Autodesk Inventor part; units mm, degrees
ref_plane "YZ Plane" through (0, 0, 0) normal (1, 0, 0) x (0, 1, 0)
ref_plane "XZ Plane" through (0, 0, 0) normal (0, 1, 0) x (-1, 0, 0)
ref_plane "XY Plane" through (0, 0, 0) normal (0, 0, 1) x (1, 0, 0)
sketch "Skizze1" plane through (0, 0, 0) normal (0, 0, 1) x (1, 0, 0)
  line L0 (-3.175, -3.175) -> (3.175, -3.175)
  line L1 (3.175, -3.175) -> (3.175, 3.175)
  line L2 (3.175, 3.175) -> (-3.175, 3.175)
  line L3 (-3.175, 3.175) -> (-3.175, -3.175)
  line L4 (-3.175, -3.175) -> (3.175, 3.175) construction
  line L5 (3.175, -3.175) -> (-3.175, 3.175) construction
  point P0 (0, 0)
  dimension "d0" = 6.35
  dimension "d1" = 6.35
extrude "Extrusion1" add sketch "Skizze1" along normal blind 1.65
sketch "Skizze2" plane through (0, 0, 1.65) normal (0, 0, 1) x (1, 0, 0)
  circle A0 centre (0, 0) radius 3.175
  dimension "d4" = 6.35
extrude "Extrusion2" add sketch "Skizze2" along normal blind 7.87
sketch "Skizze3" plane through (0, 0, 9.52) normal (0, 0, 1) x (1, 0, 0)
  circle A0 centre (0, 0) radius 2.155
  dimension "d7" = 4.31
extrude "Extrusion3" cut sketch "Skizze3" against normal blind 2
sketch "Skizze4" plane through (0, 0, 7.52) normal (0, 0, 1) x (1, 0, 0)
  circle A0 centre (0, 0) radius 0.38
  dimension "d10" = 0.76
extrude "Extrusion4" cut sketch "Skizze4" against normal blind 5
thread "Gewinde1"
sketch "Skizze5" plane through (0, 0, 0) normal (0, 0, -1) x (-1, 0, 0)
  circle A0 centre (0, 0) radius 0.5
  dimension "d15" = 1
extrude "Extrusion5" add sketch "Skizze5" along normal blind 3.81
sketch "Skizze6" plane through (0, 0, 0) normal (0, 0, -1) x (-1, 0, 0)
  line L0 (0, -4.445) -> (0, 4.445)
  line L1 (3.175, 3.175) -> (3.175, 0)
  arc A0 (-3.175, 0) -> (0, -3.175) centre (0, 0) ccw
  line L2 (3.175, 3.175) -> (2.105, 3.175)
  line L3 (2.105, 3.175) -> (2.105, 2.105)
  line L4 (2.105, 2.105) -> (3.175, 2.105)
  line L5 (3.175, 2.105) -> (3.175, 3.175)
  line L6 (-3.175, 3.175) -> (-2.105, 3.175)
  line L7 (-2.105, 3.175) -> (-2.105, 2.105)
  line L8 (-2.105, 2.105) -> (-3.175, 2.105)
  line L9 (-3.175, 2.105) -> (-3.175, 3.175)
  line L10 (-3.175, 3.175) -> (3.175, 3.175)
  line L11 (3.175, 0.375) -> (2.155, 0.375)
  line L12 (2.155, 0.375) -> (2.155, -0.645)
  line L13 (2.155, -0.645) -> (3.175, -0.645)
  line L14 (3.175, -0.645) -> (3.175, 0.375)
  line L15 (-3.175, -3.175) -> (-3.175, 3.175)
  line L16 (-3.175, 0.375) -> (-2.155, 0.375)
  line L17 (-2.155, 0.375) -> (-2.155, -0.645)
  line L18 (-2.155, -0.645) -> (-3.175, -0.645)
  line L19 (-3.175, -0.645) -> (-3.175, 0.375)
  dimension "d22" = 1.07
  dimension "d23" = 1.07
  dimension "d24" = 1.07
  dimension "d25" = 1.07
  dimension "d28" = 1.02
  dimension "d29" = 1.02
  dimension "d30" = 1.02
  dimension "d31" = 1.02
  dimension "d32" = 1.73
extrude "Extrusion6" add sketch "Skizze6" along normal blind 3.81 contours L1 L14 L13 L12 L11 | L2 L1 L4 L3 | L18 L15 A0 | A0 L15 L16 L17 L18 | L7 L8 L9 L6
properties part number "CON-SMA-EDGE-S" material "Messing, weicher Gelbton"
Check sheet for the modelled part. Datum: model origin and axes. Units: mm. A direction names the side the tool comes from. Round coordinates to 2 decimals unless told otherwise and drop trailing zeros. Loops run counter-clockwise (first coordinate to the right, second up) from the corner with the lowest first, then second, coordinate; pieces in that order, holes last. Notation, with made-up numbers: M 48.5,63.5 L 83.5,63.5 A6 ccw 83.5,73.5 Z; hole C 43.25,41.5 d8. An arc over 180 degrees is marked long. One line per question, with ' | ' between items. Start each with the question number.
Item 1: Section check A-A (z = -2.5). Record the boundary of the cut face in (x, y) (3 decimals), and give its area (3 significant figures).
Item 2: Section check C-C (x = -1). Record the boundary of the cut face in (y, z) (3 decimals), and give its area (3 significant figures).
Item 3: Section check D-D (z = 5.5). Record the boundary of the cut face in (x, y) (3 decimals).
Item 4: Gauge pin test, flat ends, axial feed: pin 1 Ø0.9 at (x, z) = (2.5, -3) entering from -Y (3 decimals); pin 2 Ø3.5 at (x, y) = (1, -1.5) entering from +Z. Record the tip position at first contact, or that the pin passes through.
Item 5: Scan lines: probe 1 along Y at (x, z) = (0, 4.9) (3 decimals); probe 2 along Y at (x, z) = (0, 8.25) (3 decimals); probe 3 along Z at (x, y) = (-1, 1.25). Record each from-to range of solid material in increasing order.
Item 6: Section check B-B (y = 0.75). Record the boundary of the cut face in (x, z) (3 decimals).
Item 7: Set-up check for faces 1 (the face through (3, 0.375, -2)), 2 (the face through (3, -3, 1.65)), 3 (the face through (-1.71, -1.31, 8.53)), 4 (the face through (-3, -2, 1.65)), 5 (the face through (3, 2.105, -2)): record each of +Z, -Z, +X, -X, +Y, -Y from which the full face is reachable in a straight line by a thin tool's end or side.
Item 8: Release check for a two-part mould opening along X. For faces 6 (the face through (0.108, 0.488, -1.878)), 7 (the face through (-3.175, 0, -1)), 8 (the face through (-3, 2.105, -2)), 9 (the face through (-2.155, 0, -2)) record: released by +X, released by -X, zero draft, split by the parting line, or undercut.
Worked out:
1) outline: M -3.175,-0.645 L -2.155,-0.645 L -2.155,0.375 L -3.175,0.375 Z; M -3.175,2.105 L -2.105,2.105 L -2.105,3.175 L -3.175,3.175 Z; C 0,0 d1; M 2.105,2.105 L 3.175,2.105 L 3.175,3.175 L 2.105,3.175 Z; M 2.155,-0.645 L 3.175,-0.645 L 3.175,0.375 L 2.155,0.375 Z | area: 5.16 mm^2
2) outline: M -3.175,0 L 3.175,0 L 3.175,1.65 L 3.013,1.65 L 3.013,9.52 L 1.909,9.52 L 1.909,7.52 L -1.909,7.52 L -1.909,9.52 L -3.013,9.52 L -3.013,1.65 L -3.175,1.65 Z | area: 50.3 mm^2
3) outline: C 0,0 d6.35; hole C 0,0 d0.76
4) pin 1: y = -0.645 | pin 2: z = 9.52
5) probe 1: -3.175 to -0.38, 0.38 to 3.175 | probe 2: -3.175 to -2.155, 2.155 to 3.175 | probe 3: 0 to 7.52
6) outline: M -3.175,0 L 3.175,0 L 3.175,1.65 L 3.085,1.65 L 3.085,9.52 L 2.02,9.52 L 2.02,7.52 L -2.02,7.52 L -2.02,9.52 L -3.085,9.52 L -3.085,1.65 L -3.175,1.65 Z
7) face 1: -Z, +X | face 2: +Z, +X, -Y | face 3: +Z | face 4: +Z, -X, -Y | face 5: -Z, +X, -X
8) face 6: undercut | face 7: released by -X | face 8: zero draft | face 9: undercut
